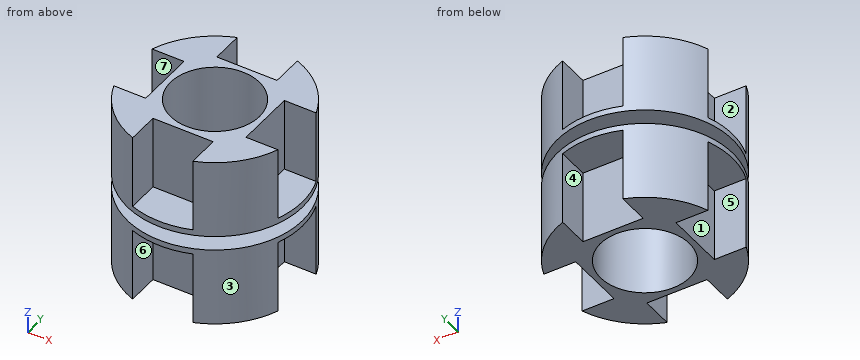
from build123d import *

# Parameters (mm, degrees)
F4_W            = 21
F4_H            = 25.5
F6_DEPTH        = 13.001
F6_COPIES_COUNT = 4


# Not quite as in the source:
# - a pattern or mirror of a feature is missing from the dataset's text; its kind, count and spacing are read off the source's solid


with BuildPart() as f5:
    # F2 (on Front) → F5 (revolve)
    with BuildSketch(Plane.XZ):
        Polygon((15.5, 30), (15.5, 0), (17.5, 0), (17.5, 2.5), (30.5, 2.5), (30.5, 30), align=None)
    revolve(axis=Axis((0, 0, 6.4842129506), (0, 0, -1)))

    # F4 (on offset) → F6 (cut, through all)
    with BuildSketch(Plane.YZ.offset(17.5)):
        with Locations((0, 17.25)):
            Rectangle(F4_W, F4_H)
    f6 = extrude(amount=F6_DEPTH, mode=Mode.SUBTRACT)

    # F6_copies: F6 ×4 about axis
    f6_copies_axis = Axis((0, 0, 0), (0, 0, 1))
    for i in range(1, F6_COPIES_COUNT):
        add(f6.rotate(f6_copies_axis, i * 360 / F6_COPIES_COUNT), mode=Mode.SUBTRACT)

    # F7: F5 across plane


with BuildPart() as f5_1:
    add(f5.part)
    add(f5.part.mirror(Plane.XY))


solid = f5_1.part
The model under review builds one solid part; all positions refer to its coordinate system, in mm. Face numbers are marked on the shaded views. A direction names the side the tool comes from. Round coordinates to 2 decimals unless told otherwise and drop trailing zeros. Write each loop counter-clockwise with the first axis right and the second up, starting at its lowest first coordinate (ties: lowest second). Pieces come first, ordered by that corner, then holes. Notation, with made-up numbers: (11.5, 5) - (62.5, 5) arc R7 cw to (62.5, 13) - close; hole circle Ø7 at (-23.75, -18). An arc over 180 degrees is marked (long way). One line per item, written item: value. Start each with the question number.
1. Machinability: for the marked faces 5, 6 and 7, which of the approach directions +Z, -Z, +X, -X, +Y, -Y give a long, thin tool a straight path to every point of the face, cutting with its end or side? Answer none if there is none.
2. Consider section A-A on x = 0. Write out the cut boundary in (y, z).
3. To check wall thickness, follow L1, parallel to Y at x = 0, z = -9; L2, parallel to Z at x = 26, y = 12.5. State the ranges of each line that lie inside material, in increasing order. Write a range as from..to.
4. The part is to be moulded in two halves that separate along Y. For the marked faces 1, 2, 3 and 4, say which applies: released by +Y, released by -Y, zero draft, split by the parting line, or undercut.
5. Consider section B-B on y = 1. Write out the cut boundary in (x, z), and give its area (3 significant figures).
6. Clearance check with flat-ended pins moving along their axes: P1, Ø6.5, axis at x = 2.5, z = 18.5, coming from the +Y side; P2, Ø8, axis at x = 5.5, z = 10.5, coming from the -Y side; P3, Ø5.5, axis at y = -25.5, z = -15, coming from the -X side. State where each tip first meets the part, or that it passes through.
7. Consider section C-C on z = 11. Write out the cut boundary in (x, y).
8. Consider section D-D on x = 21.5. Write out the cut boundary in (y, z).
Checks:
1. face 5: -Z, -X
1. face 6: -Z, -Y
1. face 7: +Z, -X
2. outline: (-30.5, -4.5) - (-17.5, -4.5) - (-17.5, -30) - (-15.5, -30) - (-15.5, 30) - (-17.5, 30) - (-17.5, 4.5) - (-30.5, 4.5) - (-30.5, 2.5) - (-17.5, 2.5) - (-17.5, -2.5) - (-30.5, -2.5) - close; (15.5, -30) - (17.5, -30) - (17.5, -4.5) - (30.5, -4.5) - (30.5, -2.5) - (17.5, -2.5) - (17.5, 2.5) - (30.5, 2.5) - (30.5, 4.5) - (17.5, 4.5) - (17.5, 30) - (15.5, 30) - close
3. L1: y = -17.5..-15.5, 15.5..17.5
3. L2: z = -30..-2.5, 2.5..30
4. face 1: undercut
4. face 2: undercut
4. face 3: split by the parting line
4. face 4: zero draft
5. outline: (-30.48, -4.5) - (-17.5, -4.5) - (-17.5, -30) - (-15.47, -30) - (-15.47, 30) - (-17.5, 30) - (-17.5, 4.5) - (-30.48, 4.5) - (-30.48, 2.5) - (-17.47, 2.5) - (-17.47, -2.5) - (-30.48, -2.5) - close; (15.47, -30) - (17.5, -30) - (17.5, -4.5) - (30.48, -4.5) - (30.48, -2.5) - (17.47, -2.5) - (17.47, 2.5) - (30.48, 2.5) - (30.48, 4.5) - (17.5, 4.5) - (17.5, 30) - (15.47, 30) - close
5. area: 347 mm^2
6. P1: stops at y = 17.5
6. P2: stops at y = -17.5
6. P3: stops at x = -20.31
7. outline: (-28.64, -10.5) arc R30.5 ccw to (-10.5, -28.64) - (-10.5, -17.5) - (10.5, -17.5) - (10.5, -28.64) arc R30.5 ccw to (28.64, -10.5) - (17.5, -10.5) - (17.5, 10.5) - (28.64, 10.5) arc R30.5 ccw to (10.5, 28.64) - (10.5, 17.5) - (-10.5, 17.5) - (-10.5, 28.64) arc R30.5 ccw to (-28.64, 10.5) - (-17.5, 10.5) - (-17.5, -10.5) - close; hole circle Ø31 at (0, 0)
8. outline: (-21.63, -30) - (-10.5, -30) - (-10.5, -4.5) - (10.5, -4.5) - (10.5, -30) - (21.63, -30) - (21.63, -2.5) - (-21.63, -2.5) - close; (-21.63, 2.5) - (21.63, 2.5) - (21.63, 30) - (10.5, 30) - (10.5, 4.5) - (-10.5, 4.5) - (-10.5, 30) - (-21.63, 30) - close
